from build123d import *

# Parameters (mm, degrees)
SKETCH1_W           = 20
SKETCH1_H           = 20
BOSS_EXTRUDE1_DEPTH = 3
BOSS_EXTRUDE2_DEPTH = 5


with BuildPart() as part:
    # Sketch1 → Boss-Extrude1 (new body)
    with BuildSketch(Plane.XY):
        with Locations((10, 10)):
            Rectangle(SKETCH1_W, SKETCH1_H)
    extrude(amount=BOSS_EXTRUDE1_DEPTH)

    # Sketch2 → Boss-Extrude2 (add)
    with BuildSketch(Plane.XY.offset(3)):
        Polygon((6.9, 20), (6.9, 18.4), (5.9, 18.4), (5.9, 16.4), (13.1, 16.4), (14.1, 16.4), (14.1, 18.4), (13.1, 18.4), (13.1, 20), align=None)
    extrude(amount=BOSS_EXTRUDE2_DEPTH)


solid = part.part
Geometry check sheet. Reference: the model listing, model coordinates, mm. A direction names the side the tool comes from. Coordinates: 2 decimals unless noted, no trailing zeros. Order: outer loops, then holes, each group sorted by start corner. A loop starts at its lowest first (then second) coordinate and runs counter-clockwise, first axis right, second up. Notation, with made-up numbers: (-37, 64.25) -> (3, 64.25) arc R17 ccw to (3, 88.25) -> close; hole circle Ø3 at (53.25, 35.5). An arc over 180 degrees is marked (long way). Use a Markdown table: item, result. Add a question column.
1. Cross-section at A-A (x = 6.5). Enter the section's corners in (y, z), and give its area (3 significant figures).
2. Set-up check for faces 1 (the face through (10, 16.4, 5)), 2 (the face through (13.1, 19, 5)), 3 (the face through (14.1, 17, 5)): record each of +Z, -Z, +X, -X, +Y, -Y from which the full face is reachable in a straight line by a thin tool's end or side.
3. Cross-section at B-B (y = 18). Enter the section's corners in (x, z).
4. Material ranges on L1, parallel to Z at x = 1.75, y = 9.75; L2, parallel to Y at x = 7, z = 5.5; L3, parallel to X at y = 17.25, z = 5.5, recorded low to high.
5. Cross-section at C-C (x = 12.25). Enter the section's corners in (y, z).
6. Go/stop test with flat-tipped pins: pin 1 Ø1.6 at (y, z) = (17, 6.5) entering from -X; pin 2 Ø3 at (x, y) = (6.5, 3) entering from +Z; pin 3 Ø0.8 at (y, z) = (19, 5) entering from +X; pin 4 Ø1 at (y, z) = (13.5, 5) entering from -X. Record where each tip stops, or that it passes through.
7. Cross-section at D-D (y = 12). Enter the section's corners in (x, z).
Filled sheet:
| question | item | result |
|---|---|---|
| 1 | outline | (0, 0) -> (20, 0) -> (20, 3) -> (18.4, 3) -> (18.4, 8) -> (16.4, 8) -> (16.4, 3) -> (0, 3) -> close |
| 1 | area | 70.0 mm2 |
| 2 | face 1 | +Z, +X, -X, -Y |
| 2 | face 2 | +Z, +X, +Y |
| 2 | face 3 | +Z, +X, +Y, -Y |
| 3 | outline | (0, 0) -> (20, 0) -> (20, 3) -> (14.1, 3) -> (14.1, 8) -> (5.9, 8) -> (5.9, 3) -> (0, 3) -> close |
| 4 | L1 | 0 to 3 |
| 4 | L2 | 16.4 to 20 |
| 4 | L3 | 5.9 to 14.1 |
| 5 | outline | (0, 0) -> (20, 0) -> (20, 8) -> (16.4, 8) -> (16.4, 3) -> (0, 3) -> close |
| 6 | pin 1 | x = 5.9 |
| 6 | pin 2 | z = 3 |
| 6 | pin 3 | x = 13.1 |
| 6 | pin 4 | through |
| 7 | outline | (0, 0) -> (20, 0) -> (20, 3) -> (0, 3) -> close |
